Geometry check sheet. Reference: the model listing, model coordinates, mm. A direction names the side the tool comes from. Round coordinates to 2 decimals unless told otherwise and drop trailing zeros. Write each loop counter-clockwise with the first axis right and the second up, starting at its lowest first coordinate (ties: lowest second). Pieces come first, ordered by that corner, then holes. Notation, with made-up numbers: (55, -33) - (74, -33) arc R21 cw to (74, -25) - close; hole circle Ø4 at (2.5, 36.5). An arc over 180 degrees is marked (long way). Return JSON: item names as keys, results as strings.
Autodesk Inventor part; units mm, degrees
ref_plane "YZ Plane" through (0, 0, 0) normal (1, 0, 0) x (0, 1, 0)
ref_plane "XZ Plane" through (0, 0, 0) normal (0, 1, 0) x (-1, 0, 0)
ref_plane "XY Plane" through (0, 0, 0) normal (0, 0, 1) x (1, 0, 0)
sketch "Sketch1" plane through (0, 0, 0) normal (0, 1, 0) x (-1, 0, 0)
  line L0 (176.1109, -25.4) -> (-176.1109, -25.4)
  line L1 (-176.1109, -25.4) -> (-176.1109, 25.4)
  line L2 (-176.1109, 25.4) -> (176.1109, 25.4)
  line L3 (176.1109, 25.4) -> (176.1109, -25.4)
  line L4 (176.1109, -25.4) -> (-176.1109, 25.4) construction
  line L5 (-176.1109, -25.4) -> (176.1109, 25.4) construction
  point P0 (0, 0)
  dimension "d0" = 352.2218
  dimension "d1" = 50.8
extrude "Extrusion1" add sketch "Sketch1" along normal blind 25.4
sketch "Sketch2" plane through (176.1109, 0, 25.4) normal (1, 0, 0) x (0, 0, -1)
  line L0 (25.4, 0) -> (25.4, 12.7) construction
  line L1 (1.5875, 23.8125) -> (49.2125, 23.8125)
  line L2 (49.2125, 23.8125) -> (49.2125, 1.5875)
  line L3 (49.2125, 1.5875) -> (1.5875, 1.5875)
  line L4 (1.5875, 1.5875) -> (1.5875, 23.8125)
  line L5 (1.5875, 23.8125) -> (49.2125, 1.5875) construction
  line L6 (49.2125, 23.8125) -> (1.5875, 1.5875) construction
  dimension "d4" = 12.7
  dimension "d5" = 47.625
  dimension "d6" = 22.225
extrude "Extrusion2" cut sketch "Sketch2" against normal through all
sketch "Sketch3" plane through (0, 25.4, 0) normal (0, 1, 0) x (1, 0, 0)
  line L0 (-180.7718, 12.7) -> (-171.45, 12.7) construction
  line L1 (-171.45, 12.7) -> (-171.45, -12.7) construction
  line L2 (-171.45, -12.7) -> (-180.7718, -12.7) construction
  line L3 (-180.7718, -12.7) -> (-180.7718, 12.7) construction
  line L4 (-176.1109, 23.8125) -> (-176.1109, -23.8125) construction
  line L5 (-180.7718, 12.7) -> (-171.45, -12.7) construction
  line L6 (-171.45, 12.7) -> (-180.7718, -12.7) construction
  circle A0 centre (-171.45, 12.7) radius 3.175
  circle A1 centre (-171.45, -12.7) radius 3.175
  line L7 (0, 0) -> (0, -23.8125) construction
  circle A2 centre (171.45, 12.7) radius 3.175
  circle A3 centre (171.45, -12.7) radius 3.175
  point P0 (-176.1109, 0)
  dimension "d9" = 9.3218
  dimension "d10" = 25.4
  dimension "d11" = 6.35
  dimension "d12" = 6.35
extrude "Extrusion3" cut sketch "Sketch3" against normal through all
properties part number "Tube"
(1) Material ranges on line 1 along X through (y, z) = (24.9, 12.7) (3 decimals); line 2 along Z through (x, y) = (171.45, 24.9) (3 decimals); line 3 along Y through (x, z) = (111, -15), recorded low to high. Write a range as [from, to].
Response values:
{"line 1": "x = [-176.111, -174.625], [-168.275, 168.275], [174.625, 176.111]", "line 2": "z = [-25.4, -15.875], [-9.525, 9.525], [15.875, 25.4]", "line 3": "y = [0, 1.59], [23.81, 25.4]"}
(2) Section check B-B, the plane z = 12.7. Enter the section's corners in (x, y) (1 decimal).
Response values:
{"outline": "(-176.1, 0) - (-174.6, 0) - (-174.6, 1.6) - (-176.1, 1.6) - close; (-176.1, 23.8) - (-174.6, 23.8) - (-174.6, 25.4) - (-176.1, 25.4) - close; (-168.3, 0) - (168.3, 0) - (168.3, 1.6) - (-168.3, 1.6) - close; (-168.3, 23.8) - (168.3, 23.8) - (168.3, 25.4) - (-168.3, 25.4) - close; (174.6, 0) - (176.1, 0) - (176.1, 1.6) - (174.6, 1.6) - close; (174.6, 23.8) - (176.1, 23.8) - (176.1, 25.4) - (174.6, 25.4) - close"}
(3) Gauge pin test, flat end, axial feed: pin 1 (5 mm diameter, centred on x = 171.45, z = -12.7, fed in from -Y). Record the tip position at first contact, or that the pin passes through.
Response values:
{"pin 1": "passes through"}
(4) Section check D-D, the plane x = 81. Enter the section's corners in (y, z), plus the area to 3 significant figures.
Response values:
{"outline": "(0, -25.4) - (25.4, -25.4) - (25.4, 25.4) - (0, 25.4) - close; hole (1.59, -23.81) - (23.81, -23.81) - (23.81, 23.81) - (1.59, 23.81) - close", "area": "232 mm^2"}
(5) Section check A-A, the plane y = 6.25. Enter the section's corners in (x, z).
Response values:
{"outline": "(-176.11, -25.4) - (176.11, -25.4) - (176.11, -23.81) - (-176.11, -23.81) - close; (-176.11, 23.81) - (176.11, 23.81) - (176.11, 25.4) - (-176.11, 25.4) - close"}
(6) Section check C-C, the plane x = -171.45. Enter the section's corners in (y, z) (1 decimal).
Response values:
{"outline": "(0, -25.4) - (25.4, -25.4) - (25.4, -15.9) - (23.8, -15.9) - (23.8, -23.8) - (1.6, -23.8) - (1.6, -15.9) - (0, -15.9) - close; (0, -9.5) - (1.6, -9.5) - (1.6, 9.5) - (0, 9.5) - close; (0, 15.9) - (1.6, 15.9) - (1.6, 23.8) - (23.8, 23.8) - (23.8, 15.9) - (25.4, 15.9) - (25.4, 25.4) - (0, 25.4) - close; (23.8, -9.5) - (25.4, -9.5) - (25.4, 9.5) - (23.8, 9.5) - close"}
(7) Access from +Z, -Z, +X, -X, +Y, -Y to the whole of each face (thin tool, end or side, straight path). Record for faces 4 (the face through (-176.111, 24, 2)), 5 (the face through (2, 23.812, 0)).
Response values:
{"face 4": "+Z, -Z, -X, +Y, -Y", "face 5": "+X, -X"}
(8) Release check for a two-part mould opening along Y. For faces 1 (the face through (-168.52, 24.62, 13.92)), 2 (the face through (2, 25.4, 0)), 3 (the face through (2, 13, 23.812)) record: pulls with the +Y half, pulls with the -Y half, needs draft (parallel to the pull), parting line crosses it, or undercut.
Response values:
{"face 1": "needs draft", "face 2": "pulls with the +Y half", "face 3": "undercut"}
